Verification items for the finished model (mm, model axes). Face numbers are marked on the shaded views. A direction names the side the tool comes from. Round coordinates to 2 decimals unless told otherwise and drop trailing zeros. Loops run counter-clockwise (first coordinate to the right, second up) from the corner with the lowest first, then second, coordinate; pieces in that order, holes last. Notation, with made-up numbers: (58, 74) -> (79, 74) arc R19 cw to (79, 85) -> close; hole circle Ø1 at (16, 44.5). An arc over 180 degrees is marked (long way). Write item = value, one per line.
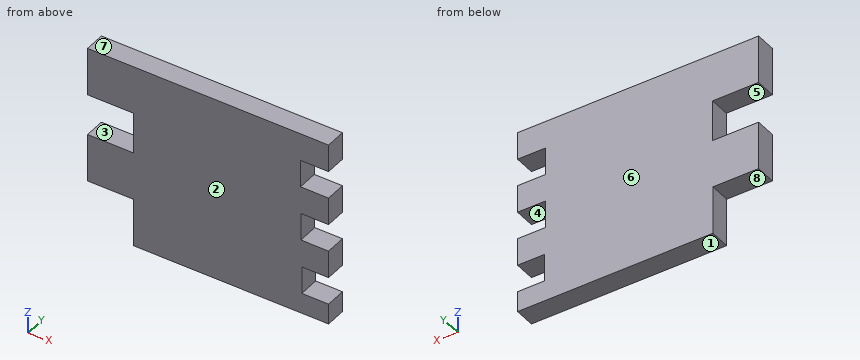
```python
from build123d import *

# Parameters (mm, degrees)
F0_W     = 175
F0_H     = 135
F1_DEPTH = 15
F2_W     = 33.1738661975
F2_H     = 35
F2_W_2   = 33.4070246667
F2_H_2   = 30
F3_DEPTH = 15.001
F4_W     = 20.4337459058
F4_H     = 20
F4_W_2   = 20.1040055603
F4_W_3   = 19.4445397705
F5_DEPTH = 15.001


with BuildPart() as f1:
    # F0 (on Front) → F1 (new body)
    with BuildSketch(Plane.XZ):
        with Locations((2.9073413461, 9.0749097914)):
            Rectangle(F0_W, F0_H)
    extrude(amount=-F1_DEPTH)

    # F2 (on face) → F3 (cut, through all)
    with BuildSketch(Plane.XZ):
        with Locations((-68.0057255551, -40.9250902086)):
            Rectangle(F2_W, F2_H)
        with Locations((-67.8891463205, 26.5749097914)):
            Rectangle(F2_W_2, F2_H_2)
    extrude(amount=-F3_DEPTH, mode=Mode.SUBTRACT)

    # F4 (on face) → F5 (cut, through all)
    with BuildSketch(Plane.XZ):
        with Locations((80.1904683933, 46.5749097914)):
            Rectangle(F4_W, F4_H)
        with Locations((80.355338566, 6.5749097914)):
            Rectangle(F4_W_2, F4_H)
        with Locations((80.6850714609, -33.4250902086)):
            Rectangle(F4_W_3, F4_H)
    extrude(amount=-F5_DEPTH, mode=Mode.SUBTRACT)


solid = f1.part
```
(1) Sectioned sample at B-B, the plane y = 12. Record the cut outline in (x, z).
Filled sheet:
outline = (-84.59, -23.43) -> (-51.42, -23.43) -> (-51.42, -58.43) -> (90.41, -58.43) -> (90.41, -43.43) -> (70.96, -43.43) -> (70.96, -23.43) -> (90.41, -23.43) -> (90.41, -3.43) -> (70.3, -3.43) -> (70.3, 16.57) -> (90.41, 16.57) -> (90.41, 36.57) -> (69.97, 36.57) -> (69.97, 56.57) -> (90.41, 56.57) -> (90.41, 76.57) -> (-84.59, 76.57) -> (-84.59, 41.57) -> (-51.19, 41.57) -> (-51.19, 11.57) -> (-84.59, 11.57) -> close
(2) Set-up check for the marked faces 4, 5, 6, 7 and 8: record each of +Z, -Z, +X, -X, +Y, -Y from which the full face is reachable in a straight line by a thin tool's end or side.
Filled sheet:
face_4 = +X, +Y, -Y
face_5 = -X, +Y, -Y
face_6 = +Z, -Z, +X, -X, +Y
face_7 = +Z, +X, -X, +Y, -Y
face_8 = -Z, -X, +Y, -Y
(3) Go/stop test with flat-tipped pins: pin 1 Ø4.5 at (x, y) = (-63.5, 6.5) entering from -Z; pin 2 Ø7.5 at (y, z) = (11, -37) entering from +X; pin 3 Ø7.5 at (y, z) = (5, 47) entering from +X. Record where each tip stops, or that it passes through.
Filled sheet:
pin_1 = -23.43
pin_2 = 70.96
pin_3 = 69.97
(4) Draft check along Z on the marked faces 1, 2 and 3. Enter one of: released by +Z, released by -Z, zero draft, split by the parting line, or undercut.
Filled sheet:
face_1 = released by -Z
face_2 = zero draft
face_3 = undercut
(5) Sectioned sample at D-D, the plane z = 27. Record the cut outline in (x, y).
Filled sheet:
outline = (-51.19, 0) -> (90.41, 0) -> (90.41, 15) -> (-51.19, 15) -> close
(6) Sectioned sample at A-A, the plane x = -65.5. Record the cut outline in (y, z), and give its area (3 significant figures).
Filled sheet:
outline = (0, -23.43) -> (15, -23.43) -> (15, 11.57) -> (0, 11.57) -> close; (0, 41.57) -> (15, 41.57) -> (15, 76.57) -> (0, 76.57) -> close
area = 1,050 mm2
(7) Sectioned sample at C-C, the plane z = 0. Record the cut outline in (x, y), and give its area (3 significant figures).
Filled sheet:
outline = (-84.59, 0) -> (70.3, 0) -> (70.3, 15) -> (-84.59, 15) -> close
area = 2,320 mm2
(8) Material ranges on probe 1 along Z at (x, y) = (77, 2.75); probe 2 along Z at (x, y) = (-68.5, 3); probe 3 along X at (y, z) = (1.5, 3), recorded low to high. Write a range as from..to.
Filled sheet:
probe_1 = -58.43..-43.43, -23.43..-3.43, 16.57..36.57, 56.57..76.57
probe_2 = -23.43..11.57, 41.57..76.57
probe_3 = -84.59..70.3
